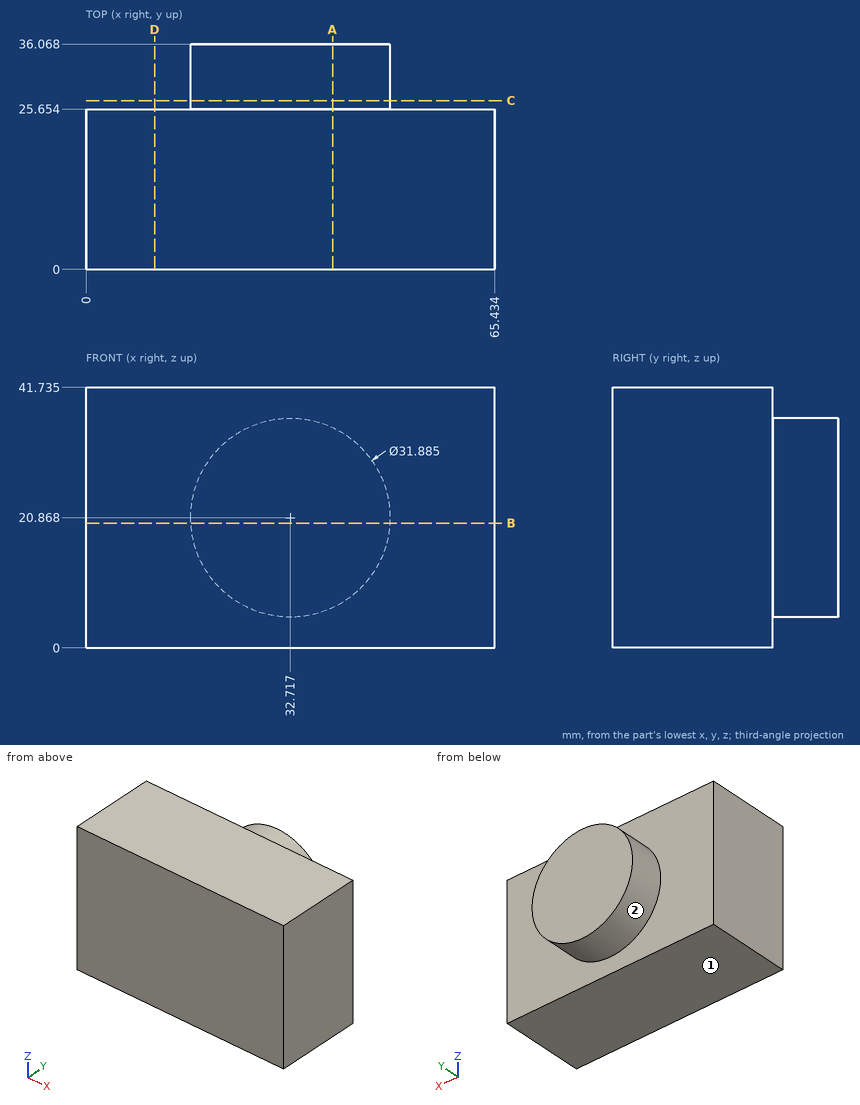
Can you work these out from the drawing? Everything is in mm from the part's minimum corner. A direction names the side the tool comes from. Give positions to 0.01 mm unless a question says otherwise; leave off trailing zeros. Loops run counter-clockwise (first coordinate to the right, second up) from the corner with the lowest first, then second, coordinate; pieces in that order, holes last. Notation, with made-up numbers: (11.25, -16.5) -> (60.25, -16.5) arc R23 ccw to (60.25, 14.5) -> close; hole circle Ø4 at (-25.5, 66). An arc over 180 degrees is marked (long way). Write item = value, one per line.
1) Suppose I cut it at A-A on x = 39.5. Write out the boundary of the cut face in (y, z) (1 decimal), then the cut area to 3 significant figures.
Check result:
outline = (0, 0) -> (25.7, 0) -> (25.7, 6.4) -> (36.1, 6.4) -> (36.1, 35.3) -> (25.7, 35.3) -> (25.7, 41.7) -> (0, 41.7) -> close
area = 1,370 mm2
2) Suppose I cut it at D-D on x = 11. Write out the boundary of the cut face in (y, z) (1 decimal).
Check result:
outline = (0, 0) -> (25.7, 0) -> (25.7, 41.7) -> (0, 41.7) -> close
3) Suppose I cut it at C-C on y = 27. Write out the boundary of the cut face in (x, z) (1 decimal).
Check result:
outline = circle Ø31.9 at (32.7, 20.9)
4) I need wall thicknesses on L1, parallel to Y at x = 44.5, z = 5; L2, parallel to X at y = 31, z = 26; L3, parallel to Z at x = 29, y = 30.5 (1 decimal). Which ranges of each line are inside material? Lowest first, please. Write a range as from..to.
Check result:
L1 = 0..25.65
L2 = 17.62..47.81
L3 = 5.4..36.4
5) For the marked faces 1 and 2, which set-ups out of +Z, -Z, +X, -X, +Y, -Y let a thin tool reach every point of the face, with its end or its side?
Check result:
face_1 = -Z, +X, -X, +Y, -Y
face_2 = +Y
6) Suppose I cut it at B-B on z = 20. Write out the boundary of the cut face in (x, y).
Check result:
outline = (0, 0) -> (65.43, 0) -> (65.43, 25.65) -> (48.64, 25.65) -> (48.64, 36.07) -> (16.8, 36.07) -> (16.8, 25.65) -> (0, 25.65) -> close
